from build123d import *

# Parameters (mm, degrees)
F1_DEPTH  = 863.6
F2_W      = 342.9
F2_H      = 622.3
F3_DEPTH  = 25.4
F4_R      = 6.35
F5_W      = 368.3
F5_H      = 635
F6_DEPTH  = 9.652
F7_R      = 6.35
F9_DEPTH  = 101.6
F10_W     = 495.3
F10_H     = 762
F10_W_2   = 469.9
F10_H_2   = 736.6
F11_DEPTH = 12.7
F12_W     = 508
F12_H     = 762
F12_W_2   = 469.9
F12_H_2   = 736.6
F13_DEPTH = 12.7


with BuildPart() as f1:
    # F0 (on Top) → F1 (new body)
    with BuildSketch(Plane.XY):
        Polygon((0, 914.4), (0, 0), (419.1, 0), (419.1, 495.3), (914.4, 495.3), (914.4, 914.4), align=None)
    extrude(amount=F1_DEPTH)

    # F2 (on face) → F3 (cut)
    with BuildSketch(Plane.YZ.offset(419.1)):
        with Locations((247.65, 476.25)):
            Rectangle(F2_W, F2_H)
    extrude(amount=-F3_DEPTH, mode=Mode.SUBTRACT)

    # F4
    f4_edges = [f1.edges().sort_by_distance(p)[0] for p in [
        (393.7, 419.1, 476.25),
        (393.7, 247.65, 787.4),
        (393.7, 76.2, 476.25),
        (393.7, 247.65, 165.1),
    ]]
    fillet(f4_edges, radius=F4_R)

    # F5 (on face) → F6 (cut)
    with BuildSketch(Plane.XZ.offset(-495.3)):
        with Locations((666.75, 482.6)):
            Rectangle(F5_W, F5_H)
    extrude(amount=-F6_DEPTH, mode=Mode.SUBTRACT)

    # F7
    f7_edges = [f1.edges().sort_by_distance(p)[0] for p in [
        (850.9, 504.952, 482.6),
        (666.75, 504.952, 800.1),
        (482.6, 504.952, 482.6),
        (666.75, 504.952, 165.1),
    ]]
    fillet(f7_edges, radius=F7_R)

    # F8 (on face) → F9 (cut)
    with BuildSketch(Plane(origin=(0, 0, 0), x_dir=(1, 0, 0), z_dir=(0, 0, -1))):
        Polygon((419.1, -495.3), (419.1, 0), (290.321976, 0), (290.321976, -613.257587), (914.4, -613.257587), (914.4, -495.3), align=None)
    extrude(amount=-F9_DEPTH, mode=Mode.SUBTRACT)

    # F10 (on face) → F11 (cut)
    with BuildSketch(Plane.YZ.offset(419.1)):
        with Locations((247.65, 482.6)):
            Rectangle(F10_W, F10_H)
        with Locations((247.65, 482.6)):
            Rectangle(F10_W_2, F10_H_2, mode=Mode.SUBTRACT)
    extrude(amount=-F11_DEPTH, mode=Mode.SUBTRACT)

    # F12 (on face) → F13 (cut)
    with BuildSketch(Plane.XZ.offset(-495.3)):
        with Locations((660.4, 482.6)):
            Rectangle(F12_W, F12_H)
        with Locations((666.75, 482.6)):
            Rectangle(F12_W_2, F12_H_2, mode=Mode.SUBTRACT)
    extrude(amount=-F13_DEPTH, mode=Mode.SUBTRACT)


solid = f1.part
Design review of the part built by this model. Coordinates are the model's own, in mm. A direction names the side the tool comes from. Round coordinates to 2 decimals unless told otherwise and drop trailing zeros. Write each loop counter-clockwise with the first axis right and the second up, starting at its lowest first coordinate (ties: lowest second). Pieces come first, ordered by that corner, then holes.
Item 1: Consider section B-B on x = 722.5. Give the boundary of the cut face in (y, z).
Item 2: Consider section D-D on x = 461. Give the boundary of the cut face in (y, z), and give its area (3 significant figures).
Item 3: For pin 1 Ø1.7 at (x, y) = (690, 496.5) entering from -Z; pin 2 Ø1 at (y, z) = (496.5, 360.5) entering from +X; pin 3 Ø1 at (y, z) = (215.5, 626.5) entering from +X, all flat-tipped, find the tip position at first contact; note any pin that passes through.
Item 4: Wall thickness on L1, parallel to Z at x = 401, y = 213; L2, parallel to X at y = 377, z = 348; L3, parallel to Z at x = 548.5, y = 536: over which ranges is each line inside the solid? List them lowest first.
Item 5: Draft analysis for pull direction X (two halves, no side actions). For faces 1 (the flat face through (349, 667, 0)), 2 (the flat face through (419.1, 36, 477)), 3 (the flat face through (664, 504.952, 487)), 4 (the flat face through (406.4, 497, 368)), state which applies: released by +X, released by -X, zero draft, split by the parting line, or undercut.
Item 6: Consider section A-A on z = 135. Give the boundary of the cut face in (x, y).
Item 7: Consider section C-C on y = 197.5. Give the boundary of the cut face in (x, z).
Item 8: For faces 5 (the flat face through (393.7, 245, 481)), 6 (the flat face through (290.322, 302, 50)), 7 (the flat face through (200, 0, 426)), 8 (the flat face through (349, 565, 863.6)), 9 (the flat face through (455, 495.3, 477)), list the 3-axis set-ups (+Z, -Z, +X, -X, +Y, -Y) from which the entire face can be reached by the end or side of a thin tool; tool diameter is ignored.
Check values:
1. outline: (495.3, 114.3) - (508, 114.3) - (508, 101.6) - (613.26, 101.6) - (613.26, 0) - (914.4, 0) - (914.4, 863.6) - (508, 863.6) - (508, 850.9) - (495.3, 850.9) - (495.3, 800.1) - (498.6, 800.1) arc R6.35 cw to (504.95, 793.75) - (504.95, 171.45) arc R6.35 cw to (498.6, 165.1) - (495.3, 165.1) - close
2. outline: (495.3, 114.3) - (508, 114.3) - (508, 101.6) - (613.26, 101.6) - (613.26, 0) - (914.4, 0) - (914.4, 863.6) - (508, 863.6) - (508, 850.9) - (495.3, 850.9) - close
2. area: 350,000 mm2
3. pin 1: stops at z = 114.3
3. pin 2: stops at x = 901.7
3. pin 3: stops at x = 393.7
4. L1: z = 101.6 to 165.1, 787.4 to 863.6
4. L2: x = 0 to 393.7
4. L3: z = 101.6 to 863.6
5. face 1: zero draft
5. face 2: released by +X
5. face 3: undercut
5. face 4: undercut
6. outline: (0, 0) - (406.4, 0) - (406.4, 12.7) - (419.1, 12.7) - (419.1, 482.6) - (406.4, 482.6) - (406.4, 508) - (431.8, 508) - (431.8, 495.3) - (901.7, 495.3) - (901.7, 508) - (914.4, 508) - (914.4, 914.4) - (0, 914.4) - close
7. outline: (0, 0) - (290.32, 0) - (290.32, 101.6) - (406.4, 101.6) - (406.4, 114.3) - (419.1, 114.3) - (419.1, 165.1) - (400.05, 165.1) arc R6.35 cw to (393.7, 171.45) - (393.7, 781.05) arc R6.35 cw to (400.05, 787.4) - (419.1, 787.4) - (419.1, 850.9) - (406.4, 850.9) - (406.4, 863.6) - (0, 863.6) - close
8. face 5: +X
8. face 6: -Z, +X, -Y
8. face 7: +Z, -Z, +X, -X, -Y
8. face 8: +Z, +X, -X, +Y, -Y
8. face 9: +Z, -Z, +X, -Y
